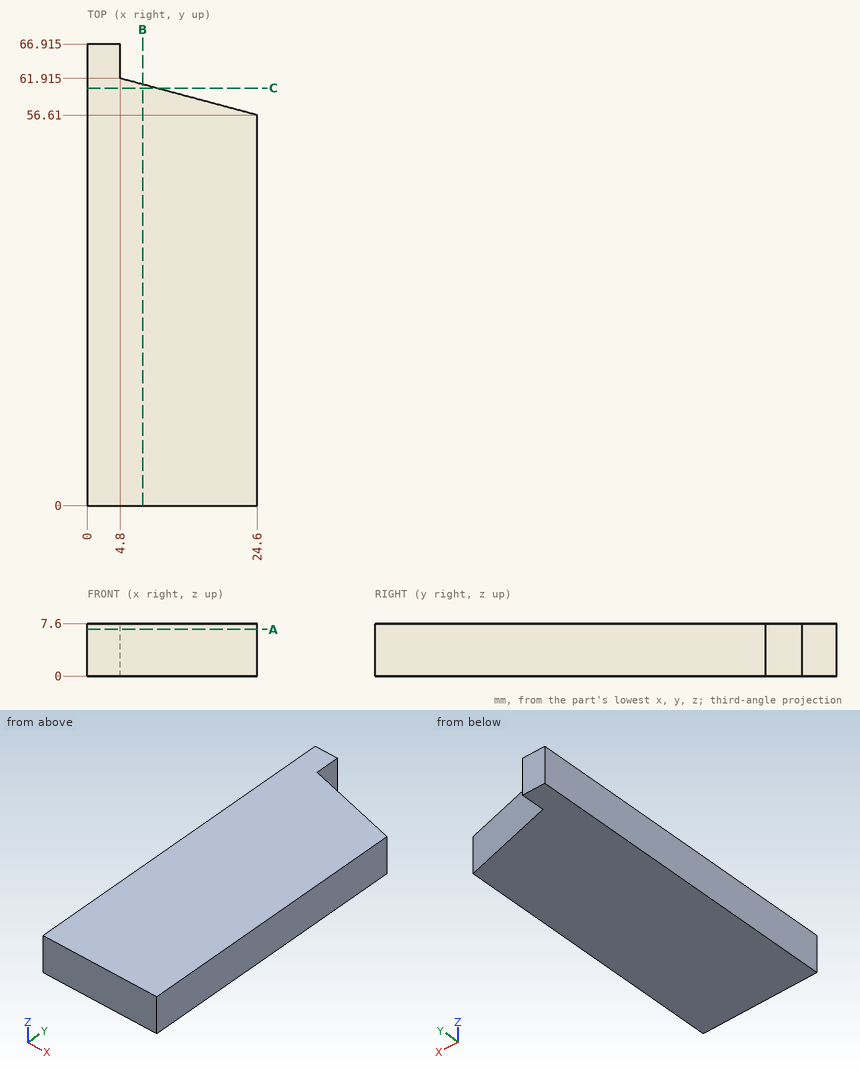
Could you check a few things on this drawing? It's one solid part, dimensions in mm from its lowest x, y, z. Coordinates: 2 decimals unless noted, no trailing zeros. Write each loop counter-clockwise with the first axis right and the second up, starting at its lowest first coordinate (ties: lowest second). Pieces come first, ordered by that corner, then holes.
1) If we section it at A-A (z = 6.75): List the corners of the cut face in (x, y) for me (1 decimal).
Filled in:
outline: (0, 0) - (24.6, 0) - (24.6, 56.6) - (4.8, 61.9) - (4.8, 66.9) - (0, 66.9) - close
2) If I drill on line 1 (Y direction, x = 9, z = 2.5); line 2 (Y direction, x = 18.5, z = 3) (1 decimal), over which ranges is the centre line in solid material (lowest first)?
Filled in:
line 1: y = 0 to 60.79
line 2: y = 0 to 58.2
3) If we section it at B-B (x = 8): List the corners of the cut face in (y, z) for me, plus the area to 3 significant figures.
Filled in:
outline: (0, 0) - (61.06, 0) - (61.06, 7.6) - (0, 7.6) - close
area: 464 mm2
4) If we section it at C-C (y = 60.5): List the corners of the cut face in (x, z) for me, plus the area to 3 significant figures.
Filled in:
outline: (0, 0) - (10.08, 0) - (10.08, 7.6) - (0, 7.6) - close
area: 76.6 mm2
5) I'm going to push a flat-ended pin straight in: pin 1 (3 mm diameter, centred on x = 20, y = 29, fed in from -Z). Where does the tip first touch, or does it pass through?
Filled in:
pin 1: stops at z = 0
